Input: dimensioned drawing with shaded views. Units: mm. Origin: part minimum x, y, z. Give positions to 0.01 mm unless a question says otherwise; leave off trailing zeros. Write each loop counter-clockwise with the first axis right and the second up, starting at its lowest first coordinate (ties: lowest second). Pieces come first, ordered by that corner, then holes. Notation, with made-up numbers: (-3, 55.5) -> (10, 55.5) arc R31 cw to (10, 83.5) -> close; hole circle Ø11 at (52, 1). An arc over 180 degrees is marked (long way). Answer as a JSON object with one key per item and string values. Group by question number.
(1) Section query A-A on y = 127. Output: boundary loops of the cut face in (x, z), plus the area to 3 significant figures.
(2) Section query D-D on y = 166.5. Output: boundary loops of the cut face in (x, z).
(3) Material intervals for probe 1 along Z at (x, y) = (6.75, 127); probe 2 along Z at (x, y) = (20.75, 196); probe 3 along Y at (x, z) = (21.25, 59.5) (1 decimal), sorted ascending.
(4) Contact query for flat-ended pins moving along their axis: pin 1 Ø2 at (x, y) = (11.5, 162) entering from -Z (1 decimal); pin 2 Ø13.5 at (y, z) = (59.65, 194.35) entering from -X; pin 3 Ø3 at (x, z) = (14, 102.5) entering from -Y; pin 4 Ø8 at (x, y) = (10, 72.5) entering from +Z. Output: stop coordinate, or through.
(5) Section query C-C on x = 5. State how many separate pieces and enclosed holes the cut face has, plus the area to 3 significant figures.
(6) Draft query along Y for the marked faces 1, 2 and 3. Return one class per face: +Y half, -Y half, draft (parallel to the pull), parting line (faces both ways), or undercut.
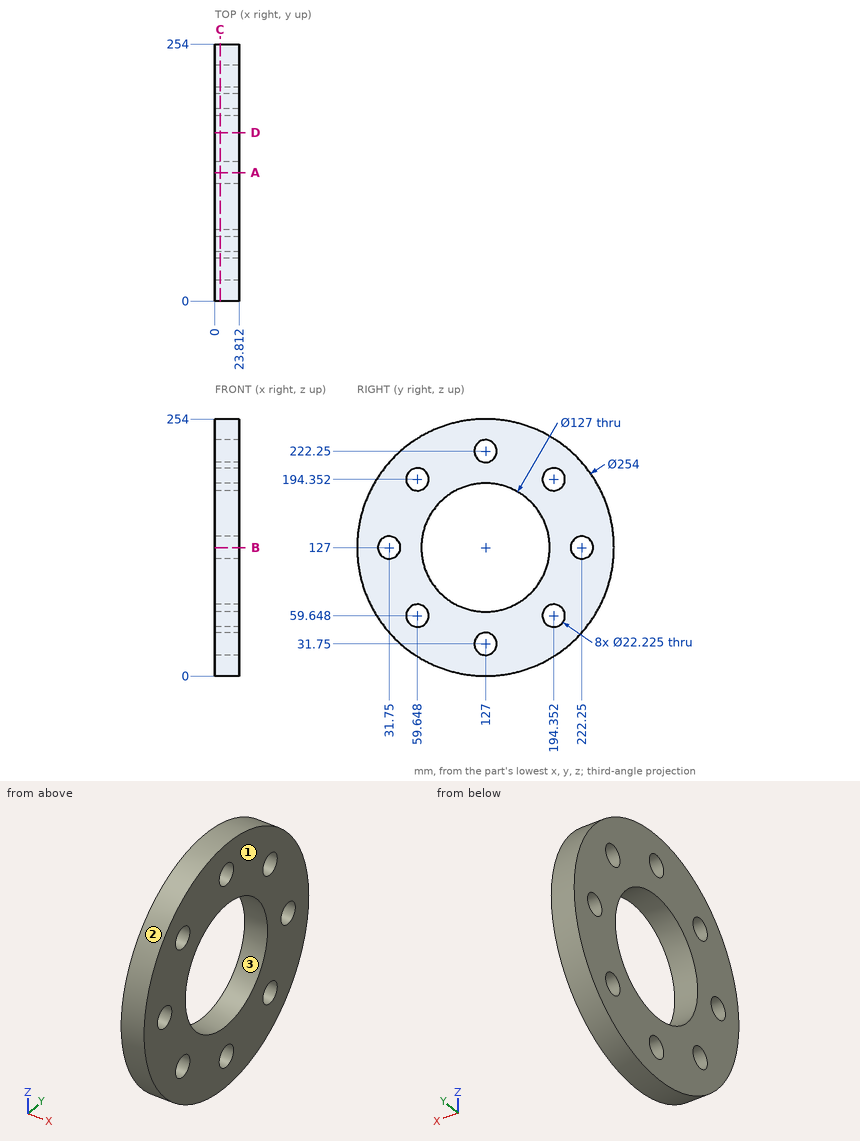
Answer list:
{
 "1": {"outline": "(0, 0) -> (23.81, 0) -> (23.81, 20.64) -> (0, 20.64) -> close; (0, 42.86) -> (23.81, 42.86) -> (23.81, 63.5) -> (0, 63.5) -> close; (0, 190.5) -> (23.81, 190.5) -> (23.81, 211.14) -> (0, 211.14) -> close; (0, 233.36) -> (23.81, 233.36) -> (23.81, 254) -> (0, 254) -> close", "area": "1,970 mm2"},
 "2": {"outline": "(0, 6.3) -> (23.81, 6.3) -> (23.81, 77.28) -> (0, 77.28) -> close; (0, 176.72) -> (23.81, 176.72) -> (23.81, 247.7) -> (0, 247.7) -> close"},
 "3": {"probe 1": "0 to 20.64, 42.86 to 63.5, 190.5 to 211.14, 233.36 to 254", "probe 2": "20.38 to 48.66, 70.64 to 183.36, 205.34 to 233.62", "probe 3": "19.4 to 48.5, 70.8 to 183.2, 205.5 to 234.6"},
 "4": {"pin 1": "z = 4.6", "pin 2": "through", "pin 3": "y = 2.1", "pin 4": "z = 243.53"},
 "5": {"separate pieces": "1", "enclosed holes": "9", "area": "34,900 mm2"},
 "6": {"face 1": "draft", "face 2": "parting line", "face 3": "undercut"}
}
